Study the drawing (mm; zero at the part's minimum x, y, z) and answer. Give positions to 0.01 mm unless a question says otherwise; leave off trailing zeros. Loops run counter-clockwise (first coordinate to the right, second up) from the corner with the lowest first, then second, coordinate; pieces in that order, holes last. Notation, with made-up numbers: M 73.5,-34 L 101.5,-34 A24 ccw 101.5,-8 Z; hole C 81,38.25 d8. An arc over 180 degrees is marked long. Return JSON: item names as keys, results as strings.
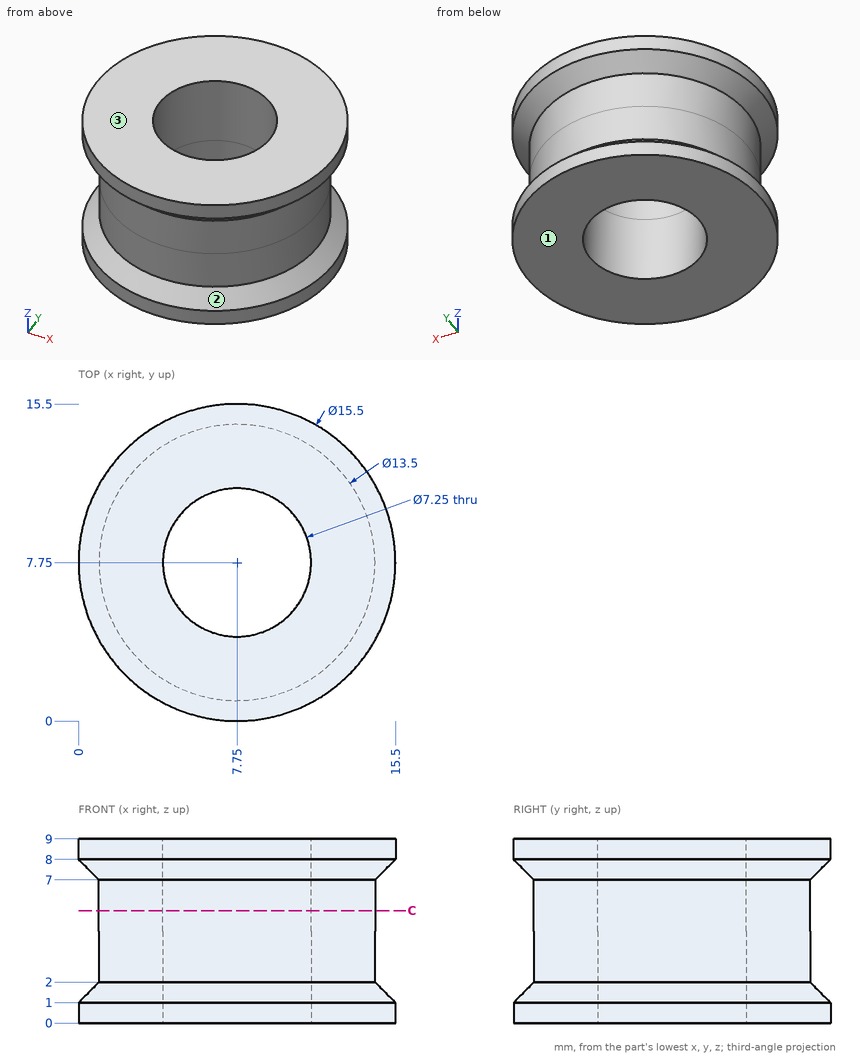
(1) Straight lines are drawn through the part: line 1 along Y through (x, z) = (7.75, 6.25) (3 decimals); line 2 along Z through (x, y) = (12.75, 2.5); line 3 along X through (y, z) = (4.5, 5) (1 decimal). For each, find the intervals that lie inside material, in ascending order.
Values follow:
{"line 1": "1 to 4.125, 11.375 to 14.5", "line 2": "0 to 1.5, 7.5 to 9", "line 3": "1.8 to 6.1, 9.4 to 13.7"}
(2) Given pin 1 (4 mm diameter, centred on x = 9.5, z = 3, fed in from +Y); pin 2 (2 mm diameter, centred on x = 3.5, z = 7, fed in from +Y); pin 3 (1 mm diameter, centred on y = 2, z = 3.5, fed in from -X), each flat-ended and moving along its own axis, determine where each tip first touches the part or whether it passes through.
Values follow:
{"pin 1": "y = 15.34", "pin 2": "y = 14.38", "pin 3": "x = 3.51"}
(3) Determine the mould class of the marked faces 1, 2 and 3 for opening direction Z: released by +Z, released by -Z, zero draft, split by the parting line, or undercut.
Values follow:
{"face 1": "released by -Z", "face 2": "undercut", "face 3": "released by +Z"}
(4) The part is cut by section C-C (z = 5.5). Determine the outline of the cut face in (x, y) (3 decimals), and give its area (3 significant figures).
Values follow:
{"outline": "C 7.75,7.75 d13.5; hole C 7.75,7.75 d7.25", "area": "102 mm²"}
